from build123d import *

# Parameters (mm, degrees)
SKETCH_1_W             = 150
SKETCH_1_H             = 80
SKETCH_1_R             = 1.3
SKETCH_1_R_2           = 22
EXTRUDE_1_DEPTH        = 5
SKETCH_2_R             = 2.34
CUT_EXTRUDE_1_DEPTH    = 2.5
SKETCH_3_R             = 1.55
SKETCH_3_R_2           = 1.582849294
CUT_EXTRUDE_3_DEPTH    = 12.5
CUT_EXTRUDE_5_DEPTH    = 8
FILLET_3_R             = 2
FILLET_3_OF_MIRROR_2_R = 2
EXTRUDE_4_DEPTH        = 5
FILLET_5_R             = 5
SKETCH_11_R            = 1.55
CUT_EXTRUDE_7_DEPTH    = 25
SKETCH_12_R            = 2.05
CUT_EXTRUDE_8_DEPTH    = 10
CUT_EXTRUDE_9_DEPTH    = 10
FILLET_6_R             = 1
EXTRUDE_5_DEPTH        = 5
CUT_EXTRUDE_START      = -10
CUT_EXTRUDE_10_DEPTH   = 10


with BuildPart() as part:
    # 草图1 → 凸台-拉伸1 (new body)
    with BuildSketch(Plane.XY):
        with Locations((-5, 0)):
            Rectangle(SKETCH_1_W, SKETCH_1_H)
        with Locations((0, -24.5)):
            Circle(SKETCH_1_R, mode=Mode.SUBTRACT)
        with Locations((-21.217622393, -12.25)):
            Circle(SKETCH_1_R, mode=Mode.SUBTRACT)
        with Locations((-21.217622393, 12.25)):
            Circle(SKETCH_1_R, mode=Mode.SUBTRACT)
        Circle(SKETCH_1_R_2, mode=Mode.SUBTRACT)
        with Locations((0, 24.5)):
            Circle(SKETCH_1_R, mode=Mode.SUBTRACT)
        with Locations((21.217622393, 12.25)):
            Circle(SKETCH_1_R, mode=Mode.SUBTRACT)
        with Locations((21.217622393, -12.25)):
            Circle(SKETCH_1_R, mode=Mode.SUBTRACT)
    extrude(amount=EXTRUDE_1_DEPTH)

    # 草图2 → 切除-拉伸1 (cut)
    with BuildSketch(Plane.XY.offset(5)):
        with Locations((-21.217622393, 12.25)):
            Circle(SKETCH_2_R)
        with Locations((0, 24.5)):
            Circle(SKETCH_2_R)
        with Locations((21.217622393, 12.25)):
            Circle(SKETCH_2_R)
        with Locations((21.217622393, -12.25)):
            Circle(SKETCH_2_R)
        with Locations((0, -24.5)):
            Circle(SKETCH_2_R)
        with Locations((-21.217622393, -12.25)):
            Circle(SKETCH_2_R)
    extrude(amount=-CUT_EXTRUDE_1_DEPTH, mode=Mode.SUBTRACT)

    # 草图3 → 切除-拉伸3 (cut)
    with BuildSketch(Plane.XY.offset(5)):
        with Locations((-70, -25)):
            Circle(SKETCH_3_R)
        with Locations((-70, -5)):
            Circle(SKETCH_3_R_2)
        with Locations((-70, 25)):
            Circle(SKETCH_3_R)
        with Locations((-70, 5)):
            Circle(SKETCH_3_R_2)
    extrude(amount=-CUT_EXTRUDE_3_DEPTH, mode=Mode.SUBTRACT)

    # 草图4 → 切除-拉伸5 (cut)
    with BuildSketch(Plane.XY.offset(5)):
        Polygon((-58, 35), (-30, 35), (-58, 11.505210327), align=None)
        Polygon((-35, 25.582872687), (-58, 6.28358117), (-35, 6.28358117), align=None)
    cut_extrude_5 = extrude(amount=-CUT_EXTRUDE_5_DEPTH, mode=Mode.SUBTRACT)

    # 圆角3
    fillet_3_edges = [part.edges().sort_by_distance(p)[0] for p in [
        (-35, 6.28358117, 2.5),
        (-58, 6.28358117, 2.5),
        (-35, 25.582872687, 2.5),
        (-30, 35, 2.5),
        (-58, 11.505210327, 2.5),
        (-58, 35, 2.5),
    ]]
    fillet(fillet_3_edges, radius=FILLET_3_R)

    # 镜向2: 切除-拉伸5 across plane
    add(cut_extrude_5.mirror(Plane.ZX), mode=Mode.SUBTRACT)

    # 圆角3 of 镜向2
    fillet_3_of_mirror_2_edges = [part.edges().sort_by_distance(p)[0] for p in [
        (-35, -6.28358117, 2.5),
        (-58, -6.28358117, 2.5),
        (-35, -25.582872687, 2.5),
        (-30, -35, 2.5),
        (-58, -11.505210327, 2.5),
        (-58, -35, 2.5),
    ]]
    fillet(fillet_3_of_mirror_2_edges, radius=FILLET_3_OF_MIRROR_2_R)

    # 草图10 → 凸台-拉伸4 (add)
    with BuildSketch(Plane.XY.offset(5)):
        Polygon((-80, -40), (-127.053079228, -7.053079228), (-80, 40), align=None)
    extrude(amount=-EXTRUDE_4_DEPTH)

    # 圆角5
    fillet_5_edges = [part.edges().sort_by_distance(p)[0] for p in [
        (-127.053079228, -7.053079228, 2.5),
    ]]
    fillet(fillet_5_edges, radius=FILLET_5_R)

    # 草图11 → 切除-拉伸7 (cut)
    with BuildSketch(Plane.XY.offset(5)):
        with Locations((-15.75, 27.279800219)):
            Circle(SKETCH_11_R)
        with Locations((15.75, 27.279800219)):
            Circle(SKETCH_11_R)
        with Locations((31.5, 0)):
            Circle(SKETCH_11_R)
        with Locations((15.75, -27.279800219)):
            Circle(SKETCH_11_R)
        with Locations((-15.75, -27.279800219)):
            Circle(SKETCH_11_R)
        with Locations((-31.5, 0)):
            Circle(SKETCH_11_R)
    extrude(amount=-CUT_EXTRUDE_7_DEPTH, mode=Mode.SUBTRACT)

    # 草图12 → 切除-拉伸8 (cut)
    with BuildSketch(Plane.XY.offset(5)):
        with Locations((35, 25)):
            Circle(SKETCH_12_R)
        with Locations((65, 25)):
            Circle(SKETCH_12_R)
        with Locations((65, -25)):
            Circle(SKETCH_12_R)
        with Locations((35, -25)):
            Circle(SKETCH_12_R)
    extrude(amount=-CUT_EXTRUDE_8_DEPTH, mode=Mode.SUBTRACT)

    # 草图13 → 切除-拉伸9 (cut)
    with BuildSketch(Plane.XY.offset(5)):
        Polygon((35, 19), (35, -19), (46.4, 0), align=None)
        Polygon((65, -19), (53.6, 0), (65, 19), align=None)
        Polygon((41, 19), (50, 4), (59, 19), align=None)
        Polygon((50, -4), (59, -19), (41, -19), align=None)
    extrude(amount=-CUT_EXTRUDE_9_DEPTH, mode=Mode.SUBTRACT)

    # 圆角6
    fillet_6_edges = [part.edges().sort_by_distance(p)[0] for p in [
        (41, 19, 2.5),
        (59, 19, 2.5),
        (50, 4, 2.5),
        (65, 19, 2.5),
        (65, -19, 2.5),
        (53.6, 0, 2.5),
        (41, -19, 2.5),
        (50, -4, 2.5),
        (59, -19, 2.5),
        (35, 19, 2.5),
        (46.4, 0, 2.5),
        (35, -19, 2.5),
    ]]
    fillet(fillet_6_edges, radius=FILLET_6_R)

    # 草图14 → 凸台-拉伸5 (add)
    with BuildSketch(Plane.XY.offset(5)):
        Polygon((-80, -40), (-65.718519933, -50), (70, -50), (70, -40), align=None)
    extrude(amount=-EXTRUDE_5_DEPTH)

    # 草图15 → 切除-拉伸10 (cut)
    with BuildSketch(Plane.XY.offset(5).offset(CUT_EXTRUDE_START)):
        with BuildLine():
            Line((-80, 40), (-122.839593994, -2.839593994))
            ThreePointArc((-122.839593994, -2.839593994), (-124.285033579, -6.810906614), (-122.17194227, -10.470888122))
            Line((-122.17194227, -10.470888122), (-80, -40))
            Line((-80, -40), (-80, 0))
            Line((-80, 0), (-80, 40))
        make_face()
    extrude(amount=CUT_EXTRUDE_10_DEPTH, mode=Mode.SUBTRACT)


solid = part.part
Model file for the job. Use its own axes, mm. A direction names the side the tool comes from. Give positions to 0.01 mm unless a question says otherwise; leave off trailing zeros. Order: outer loops, then holes, each group sorted by start corner. A loop starts at its lowest first (then second) coordinate and runs counter-clockwise, first axis right, second up. Notation, with made-up numbers: M 51.25,-0.75 L 96.25,-0.75 A19 ccw 96.25,35.25 Z; hole C 11.25,49.25 d4. An arc over 180 degrees is marked long. Put each result on its own line as item: value. Start each with the question number.
(1) Tool access for faces 3 (the face through (-20, 11, 2.5)), 4 (the face through (-58, 24, 3)), 5 (the face through (1, -50, 3)): list every direction of +Z, -Z, +X, -X, +Y, -Y with a clear straight run to the whole face (end or side of a thin tool).
(2) Pin check, flat tips, straight feed: pin 1 Ø5.5 at (x, y) = (21.22, 12.25) entering from -Z; pin 2 Ø3 at (x, y) = (0, -24.5) entering from +Z. Stop position of each tip, or through.
(3) Drill centre lines: L1, parallel to Y at x = 0, z = 3.95; L2, parallel to Y at x = -40, z = 4.15; L3, parallel to Y at x = -15.5, z = 2.3. Where is each one in solid material? Low to high. Write a range as [from, to].
(4) Band-saw the part on B-B on x = 11.5. Give the cut face in (y, z) (3 decimals), then the cut area to 3 significant figures.
(5) Band-saw the part on C-C on x = -70. Give the cut face in (y, z).
(6) Pull direction Y, two halves, no side cores. Call faces 1 (the face through (41.41, -8.32, 2.54)), 2 (the face through (-73, -44.9, 2.5)): released by +Y, released by -Y, zero draft, split by the parting line, or undercut.
(7) Band-saw the part on D-D on z = 4. Count the separate pieces of the cut face and the enclosed holes in it, then the cut area to 3 significant figures.
(8) Band-saw the part on A-A on x = -15.75. Give the cut face in (y, z).
Results below:
1. face 3: +Z
1. face 4: +Z, -Z
1. face 5: +Z, -Z, +X, -X, -Y
2. pin 1: stops at z = 0
2. pin 2: stops at z = 2.5
3. L1: y = [-50, -26.84], [-22.16, -22], [22, 22.16], [26.84, 40]
3. L2: y = [-50, -35], [-26.61, -21.39], [-6.28, 6.28], [21.39, 26.61], [35, 40]
3. L3: y = [-50, -28.81], [-25.75, -15.61], [15.61, 25.75], [28.81, 40]
4. outline: M -50,0 L -18.755,0 L -18.755,5 L -50,5 Z; M 18.755,0 L 40,0 L 40,5 L 18.755,5 Z
4. area: 262 mm2
5. outline: M -47,0 L -26.55,0 L -26.55,5 L -47,5 Z; M -23.45,0 L -6.58,0 L -6.58,5 L -23.45,5 Z; M -3.42,0 L 3.42,0 L 3.42,5 L -3.42,5 Z; M 6.58,0 L 23.45,0 L 23.45,5 L 6.58,5 Z; M 26.55,0 L 40,0 L 40,5 L 26.55,5 Z
6. face 1: undercut
6. face 2: released by -Y
7. separate pieces: 1
7. enclosed holes: 29
7. area: 9,930 mm2
8. outline: M -50,0 L -28.83,0 L -28.83,5 L -50,5 Z; M -25.73,0 L -15.36,0 L -15.36,5 L -25.73,5 Z; M 15.36,0 L 25.73,0 L 25.73,5 L 15.36,5 Z; M 28.83,0 L 40,0 L 40,5 L 28.83,5 Z
